Could you check a few things on this model? Use its own coordinates, in mm. A direction names the side the tool comes from. Give positions to 0.01 mm unless a question says otherwise; leave off trailing zeros. Order: outer loops, then holes, each group sorted by start corner. A loop starts at its lowest first (then second) coordinate and runs counter-clockwise, first axis right, second up. Notation, with made-up numbers: M 13,-6 L 40,-6 A14 cw 40,2 Z; hole C 6,22.25 d3. An arc over 180 degrees is marked long. Use a Markdown table: item, result. Add a question column.
Item 1: Suppose I cut it at A-A on x = -19.05. Write out the boundary of the cut face in (y, z), plus the area to 3 significant figures.
Item 2: I'm going to push a flat-ended pin straight in: pin 1 Ø3 at (x, z) = (-19.05, 12.7) entering from -Y. Where does the tip first touch, or does it pass through?
Item 3: If I drill on L1, parallel to Z at x = 6.35, y = 4.25; L2, parallel to X at y = 4.75, z = -12.7, over which ranges is the centre line in solid material (lowest first)? Write a range as from..to.
Item 4: Suppose I cut it at B-B on y = 5.25. Write out the boundary of the cut face in (x, z), plus the area to 3 significant figures.
Item 5: Suppose I cut it at D-D on z = -11.5. Write out the boundary of the cut face in (x, y), plus the area to 3 significant figures.
Item 6: Suppose I cut it at C-C on x = 51. Write out the boundary of the cut face in (y, z).
Item 7: If we mould it in two halves opening along Z, with no side actions, what happens to faces 3 (the face through (13, 3, -25.4)), 4 (the face through (6.903, 3.131, -10.208)), 5 (the face through (12, 3, 25.4)), 6 (the face through (31.623, 3, 0))? For each: released by +Z, released by -Z, zero draft, split by the parting line, or undercut.
Item 8: For faces 1 (the face through (44, 3, -12.764)), 2 (the face through (57.15, 3, -19)), which set-ups out of +Z, -Z, +X, -X, +Y, -Y let a thin tool reach every point of the face, with its end or its side?
from build123d import *

# Parameters (mm, degrees)
BOSS_EXTRUDE1_DEPTH    = 6.35
F_10_CLEARANCE_HOLE1_D = 5.1054
SKETCH5_W              = 25.527
SKETCH5_H              = 25.527
CUT_EXTRUDE1_DEPTH     = 63.861792847


with BuildPart() as part:
    # Sketch1 → Boss-Extrude1 (new body)
    with BuildSketch(Plane(origin=(0, 0, 0), x_dir=(1, 0, 0), z_dir=(0, 1, 0))):
        Polygon((31.75, 25.4), (57.15, 25.4), (57.15, -25.4), (31.75, -25.4), (-31.75, -25.4), (-31.75, 25.4), align=None)
    extrude(amount=BOSS_EXTRUDE1_DEPTH)

    # #10 Clearance Hole1 (through all)
    with Locations(Plane(origin=(0, 6.35, 0), x_dir=(1, 0, 0), z_dir=(0, 1, 0))):
        with Locations((-19.05, 12.7), (6.35, 12.7), (6.35, -12.7), (-19.05, -12.7)):
            Hole(F_10_CLEARANCE_HOLE1_D / 2)

    # Sketch5 → Cut-Extrude1 (cut, through all)
    with BuildSketch(Plane(origin=(0, 6.35, 0), x_dir=(1, 0, 0), z_dir=(0, 1, 0))):
        with Locations((44.3865, 0)):
            Rectangle(SKETCH5_W, SKETCH5_H)
    extrude(amount=-CUT_EXTRUDE1_DEPTH, mode=Mode.SUBTRACT)


solid = part.part
Findings below:
| question | item | result |
|---|---|---|
| 1 | outline | M 0,-25.4 L 6.35,-25.4 L 6.35,-15.25 L 0,-15.25 Z; M 0,-10.15 L 6.35,-10.15 L 6.35,10.15 L 0,10.15 Z; M 0,15.25 L 6.35,15.25 L 6.35,25.4 L 0,25.4 Z |
| 1 | area | 258 mm^2 |
| 2 | pin 1 | passes through |
| 3 | L1 | z = -25.4..-15.25, -10.15..10.15, 15.25..25.4 |
| 3 | L2 | x = -31.75..-21.6, -16.5..3.8, 8.9..31.62 |
| 4 | outline | M -31.75,-25.4 L 57.15,-25.4 L 57.15,-12.76 L 31.62,-12.76 L 31.62,12.76 L 57.15,12.76 L 57.15,25.4 L -31.75,25.4 Z; hole C -19.05,-12.7 d5.11; hole C -19.05,12.7 d5.11; hole C 6.35,-12.7 d5.11; hole C 6.35,12.7 d5.11 |
| 4 | area | 3,780 mm^2 |
| 5 | outline | M -31.75,0 L -21.3,0 L -21.3,6.35 L -31.75,6.35 Z; M -16.8,0 L 4.1,0 L 4.1,6.35 L -16.8,6.35 Z; M 8.6,0 L 31.62,0 L 31.62,6.35 L 8.6,6.35 Z |
| 5 | area | 345 mm^2 |
| 6 | outline | M 0,-25.4 L 6.35,-25.4 L 6.35,-12.76 L 0,-12.76 Z; M 0,12.76 L 6.35,12.76 L 6.35,25.4 L 0,25.4 Z |
| 7 | face 3 | released by -Z |
| 7 | face 4 | undercut |
| 7 | face 5 | released by +Z |
| 7 | face 6 | undercut |
| 8 | face 1 | +X, +Y, -Y |
| 8 | face 2 | +Z, -Z, +X, +Y, -Y |
